Could you check a few things on this model? Use its own coordinates, in mm. Face numbers are marked on the shaded views. A direction names the side the tool comes from. Give positions to 0.01 mm unless a question says otherwise; leave off trailing zeros. Loops run counter-clockwise (first coordinate to the right, second up) from the corner with the lowest first, then second, coordinate; pieces in that order, holes last.
1. For the marked faces 4, 5, 6, 7 and 8, which set-ups out of +Z, -Z, +X, -X, +Y, -Y let a thin tool reach every point of the face, with its end or its side?
2. I need wall thicknesses on line 1 along X through (y, z) = (-6.95, 0) (3 decimals); line 2 along X through (y, z) = (0, 2.35); line 3 along Y through (x, z) = (0, -0.95) (3 decimals). Which ranges of each line are inside material? Lowest first, please.
3. Thinking about a two-plate mould opening in Y: for the marked faces 1, 2 and 3, which applies, +Y half, -Y half, draft (parallel to the pull), parting line (faces both ways), or undercut?
4. Imagine slicing it at A-A (z = 0). Count the separate pieces of the cut face and the enclosed holes in it, plus the area to 3 significant figures.
5. Imagine slicing it at C-C (x = -12). List the corners of the cut face in (y, z) for me (1 decimal), plus the area to 3 significant figures.
6. Imagine slicing it at B-B (x = 15). List the corners of the cut face in (y, z) for me (1 decimal), plus the area to 3 significant figures.
7. For P1, Ø3, axis at x = 6.5, z = 0.5, coming from the +Y side; P2, Ø8.5, axis at x = 0, y = 0, coming from the +Z side; P3, Ø1.8, axis at x = -1.5, y = -1, coming from the -Z side; P4, Ø2.5, axis at x = 16, z = -0.5, coming from the +Y side, each with a flat end and sliding along its axis, tell me the tip position at first contact or that it passes through.
```python
from build123d import *

# Parameters (mm, degrees)
EXTRUDE1_DEPTH      = 2.54
EXTRUDE1_DEPTH_BACK = 2.54
SKETCH3_R           = 4.7625
SKETCH4_R           = 1.5875
CUT_EXTRUDE1_DEPTH  = 24.321126052
FILLET1_R           = 1.27
FILLET2_R           = 1.27
CHAMFER1_SIZE       = 0.127
FILLET3_R           = 0.254
CHAMFER2_SIZE       = 0.127


with BuildPart() as part:
    # Sketch3 → Extrude1 (new, two sides: drawn at the far end of the back side and taken through both)
    with BuildSketch(Plane.XY.offset(-EXTRUDE1_DEPTH_BACK)):
        with BuildLine():
            Line((9.525, 0), (9.525, -4.7625))
            Line((9.525, -4.7625), (18.25625, -4.7625))
            Line((18.25625, -4.7625), (18.25625, -9.525))
            Line((18.25625, -9.525), (-18.25625, -9.525))
            Line((-18.25625, -9.525), (-18.25625, -4.7625))
            Line((-18.25625, -4.7625), (-9.525, -4.7625))
            Line((-9.525, -4.7625), (-9.525, 0))
            ThreePointArc((-9.525, 0), (0, 9.525), (9.525, 0))
        make_face()
        Circle(SKETCH3_R, mode=Mode.SUBTRACT)
    extrude(amount=EXTRUDE1_DEPTH + EXTRUDE1_DEPTH_BACK)

    # Sketch4 → Cut-Extrude1 (cut, through all)
    with BuildSketch(Plane(origin=(0, -4.7625, 0), x_dir=(1, 0, 0), z_dir=(0, 1, 0))):
        with Locations(Location((-14.2875, 0, 0), (0, 0, 270))):
            Circle(SKETCH4_R)
        with Locations(Location((14.2875, 0, 0), (0, 0, 270))):
            Circle(SKETCH4_R)
        Polygon((-18.25625, 2.54), (-18.25625, 1.27), (-16.98625, 2.54), align=None)
        Polygon((16.98625, 2.54), (18.25625, 2.54), (18.25625, 1.27), align=None)
        Polygon((18.25625, -2.54), (18.25625, -1.27), (16.98625, -2.54), align=None)
        Polygon((-16.98625, -2.54), (-18.25625, -2.54), (-18.25625, -1.27), align=None)
    extrude(amount=-CUT_EXTRUDE1_DEPTH, mode=Mode.SUBTRACT)

    # Fillet1
    fillet1_edges = [part.edges().sort_by_distance(p)[0] for p in [
        (0, 9.525, -2.54),
        (9.525, -2.38125, -2.54),
        (9.525, -2.38125, 2.54),
        (-9.525, -2.38125, -2.54),
        (0, 9.525, 2.54),
        (-9.525, -2.38125, 2.54),
    ]]
    fillet(fillet1_edges, radius=FILLET1_R)

    # Fillet2
    # the kernel refuses this fillet: 1.27 mm, written as the material it adds along each edge
    with BuildSketch(Plane(origin=(-9.525, -4.7625, -1.27), x_dir=(0, 1, 0), z_dir=(0, 0, 1)), Plane(origin=(9.525, -4.7625, 1.27), x_dir=(0, 1, 0), z_dir=(0, 0, -1))) as fillet2_piece_1:
        with BuildLine():
            CenterArc((FILLET2_R, FILLET2_R), FILLET2_R, 180, 90)
            Line((0, FILLET2_R), (0, 0))
            Line((0, 0), (FILLET2_R, 0))
        make_face()
    extrude(amount=2.54)
    with BuildSketch(Plane(origin=(8.255, -4.7625, -1.27), x_dir=(-0.5976672776328268, 0, 0.8017442392976488), z_dir=(0.8017442392976488, 0, 0.5976672776328268))) as fillet2_piece_2_section:
        with BuildLine():
            CenterArc((1.27 + FILLET2_R, -FILLET2_R), FILLET2_R, 90, 90)
            Line((1.27 + FILLET2_R, 0), (1.27, 0))
            Line((1.27, 0), (1.27, -FILLET2_R))
        make_face()
    fillet2_piece_2 = revolve(axis=Axis((8.255, -4.7625, -1.27), (0, -1, 0)), revolution_arc=233.296989237, mode=Mode.PRIVATE)
    fillet2_piece_2 = split(fillet2_piece_2, bisect_by=Plane(origin=(9.207422318, -4.366731678, -2.54), z_dir=(0, 0, 1)), keep=Keep.TOP, mode=Mode.PRIVATE)
    add(fillet2_piece_2)
    with BuildSketch(Plane(origin=(-8.255, -4.7625, -1.27), x_dir=(0.5976672776328281, 0, 0.8017442392976479), z_dir=(-0.8017442392976479, 0, 0.5976672776328281))) as fillet2_piece_3_section:
        with BuildLine():
            CenterArc((1.27 + FILLET2_R, FILLET2_R), FILLET2_R, 180, 90)
            Line((1.27, FILLET2_R), (1.27, 0))
            Line((1.27, 0), (1.27 + FILLET2_R, 0))
        make_face()
    fillet2_piece_3 = revolve(axis=Axis((-8.255, -4.7625, -1.27), (0, 1, 0)), revolution_arc=233.296989237, mode=Mode.PRIVATE)
    fillet2_piece_3 = split(fillet2_piece_3, bisect_by=Plane(origin=(-9.207422451, -4.366732131, -2.54), z_dir=(0, 0, 1)), keep=Keep.TOP, mode=Mode.PRIVATE)
    add(fillet2_piece_3)
    with BuildSketch(Plane(origin=(8.255, -4.7625, 1.27), x_dir=(1, 0, 0), z_dir=(0, 0, -1))) as fillet2_piece_4_section:
        with BuildLine():
            CenterArc((1.27 + FILLET2_R, -FILLET2_R), FILLET2_R, 90, 90)
            Line((1.27 + FILLET2_R, 0), (1.27, 0))
            Line((1.27, 0), (1.27, -FILLET2_R))
        make_face()
    fillet2_piece_4 = revolve(axis=Axis((8.255, -4.7625, 1.27), (0, -1, 0)), revolution_arc=233.296989237, mode=Mode.PRIVATE)
    fillet2_piece_4 = split(fillet2_piece_4, bisect_by=Plane(origin=(9.207422382, -4.366731938, 2.54), z_dir=(0, 0, -1)), keep=Keep.TOP, mode=Mode.PRIVATE)
    add(fillet2_piece_4)
    with BuildSketch(Plane(origin=(-8.255, -4.7625, 1.27), x_dir=(-1, 0, 0), z_dir=(0, 0, -1))) as fillet2_piece_5_section:
        with BuildLine():
            CenterArc((1.27 + FILLET2_R, FILLET2_R), FILLET2_R, 180, 90)
            Line((1.27, FILLET2_R), (1.27, 0))
            Line((1.27, 0), (1.27 + FILLET2_R, 0))
        make_face()
    fillet2_piece_5 = revolve(axis=Axis((-8.255, -4.7625, 1.27), (0, 1, 0)), revolution_arc=233.296989237, mode=Mode.PRIVATE)
    fillet2_piece_5 = split(fillet2_piece_5, bisect_by=Plane(origin=(-9.804114567, -4.550028742, 2.54), z_dir=(0, 0, -1)), keep=Keep.TOP, mode=Mode.PRIVATE)
    add(fillet2_piece_5)

    # Chamfer1
    chamfer1_edges = [part.edges().sort_by_distance(p)[0] for p in [
        (-4.7625, 0, 2.54),
        (-4.7625, 0, -2.54),
    ]]
    chamfer(chamfer1_edges, length=CHAMFER1_SIZE)

    # Sketch5 → Revolve1 (revolve)
    with BuildSketch(Plane(origin=(0, 0, 0), x_dir=(0, 0, -1), z_dir=(1, 0, 0))):
        Polygon((-2.286, 4.7625), (-2.286, 4.1671875), (-2.54, 4.1671875), (-2.54, 2.9765625), (-2.286, 2.9765625), (-2.286, 2.38125), (2.286, 2.38125), (2.286, 2.9765625), (2.54, 2.9765625), (2.54, 4.1671875), (2.286, 4.1671875), (2.286, 4.7625), align=None)
    revolve(axis=Axis((0, 0, 0), (0, 0, 1)))

    # Fillet3
    fillet3_edges = [part.edges().sort_by_distance(p)[0] for p in [
        (0, -2.38125, -2.286),
        (0, -2.38125, 2.286),
    ]]
    fillet(fillet3_edges, radius=FILLET3_R)

    # Chamfer2
    chamfer2_edges = [part.edges().sort_by_distance(p)[0] for p in [
        (0, -4.1671875, -2.54),
        (0, -2.9765625, -2.54),
        (0, -2.9765625, 2.54),
        (0, -4.1671875, 2.54),
    ]]
    chamfer(chamfer2_edges, length=CHAMFER2_SIZE)


solid = part.part
```
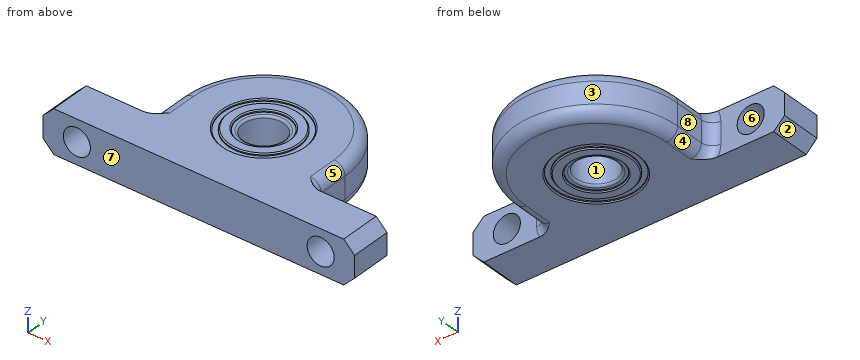
Derived:
1. face 4: -Z, -X, +Y
1. face 5: +Z, +X, +Y
1. face 6: +Y, -Y
1. face 7: +Z, -Z, +X, -X, -Y
1. face 8: +Z, -Z, -X, +Y
2. line 1: x = -18.256 to -15.875, -12.7 to 12.7, 15.875 to 18.256
2. line 2: x = -8.92 to -4.76, -4.17 to -2.98, 2.98 to 4.17, 4.76 to 8.92
2. line 3: y = -9.525 to -2.381, 2.381 to 9.525
3. face 1: undercut
3. face 2: draft
3. face 3: +Y half
4. separate pieces: 3
4. enclosed holes: 1
4. area: 360 mm2
5. outline: (-9.5, -2.5) - (-4.8, -2.5) - (-4.8, 2.5) - (-9.5, 2.5) - close
5. area: 24.2 mm2
6. outline: (-9.5, -2.5) - (-4.8, -2.5) - (-4.8, -1.4) - (-9.5, -1.4) - close; (-9.5, 1.4) - (-4.8, 1.4) - (-4.8, 2.5) - (-9.5, 2.5) - close
6. area: 10.7 mm2
7. P1: stops at y = 8.11
7. P2: stops at z = 2.54
7. P3: stops at z = -2.29
7. P4: stops at y = -4.76
